Autodesk Inventor part; units mm, degrees
ref_plane "Arbeitsebene1" through (0, 0, 0) normal (0, 1, 0) x (-1, 0, 0)
ref_plane "YZ Plane" through (0, 0, 0) normal (1, 0, 0) x (0, 1, 0)
ref_plane "XY Plane" through (0, 0, 0) normal (0, 0, 1) x (1, 0, 0)
sketch "Skizze1" plane through (0, 0, 0) normal (0, 1, 0) x (-1, 0, 0)
  circle A0 centre (0, 0) radius 75
  dimension "d0" = 150
extrude "Extrusion1" add sketch "Skizze1" along normal mid plane 6
ref_plane "Arbeitsebene1" through (0, 0, 0) normal (0, 1, 0) x (-1, 0, 0)
sketch "Skizze4" plane through (0, 0, 0) normal (0, 1, 0) x (-1, 0, 0)
  circle A0 centre (0, 0) radius 6.5
  dimension "d17" = 13
extrude "Extrusion3" add sketch "Skizze4" along normal mid plane 18
sketch "Skizze5" plane through (0, 9, 0) normal (0, 1, 0) x (1, 0, 0)
  circle A0 centre (0, 0) radius 6.5
hole "Bohrung1" at (0, 9, 0) direction (0, -1, 0) diameter 6 end up to surface
sketch "Skizze2" plane through (0, 3, 0) normal (0, 1, 0) x (1, 0, 0)
  circle A0 centre (0, 0) radius 63 construction
  circle A1 centre (0, 0) radius 75
  line L0 (0, 0) -> (0, -75) construction
  line L1 (0, 0) -> (-75, 0) construction
  circle A2 centre (0, 0) radius 6.5
  line L2 (-8, 0) -> (-54.1014, -32.2806)
  line L3 (-8, 0) -> (-54.1014, 32.2806)
  arc A3 (-54.1014, 32.2806) -> (-54.1014, -32.2806) centre (0, 0) ccw
  dimension "d3" = 126
  dimension "d40" = 8
  dimension "d41" = 35
extrude "Extrusion2" cut sketch "Skizze2" against normal up to surface (6 mm away) contours L2 A3 L3
fillet "Rundung1" radius 3 3 edges at (-8, 0, 0) (-54.1014, 0, 32.2806) (-54.1014, 0, -32.2806)
pattern_circular "Runde Anordnung3" count 5 over 360 about axis through (0, 0, 0) along (0, 1, 0) of "Extrusion2"
fillet "Rundung3" radius 3 6 edges at (24.7949, 0, -57.9156) (62.743, 0, -5.6845) (62.743, 0, 5.6845) (24.7949, 0, 57.9156) (13.9824, 0, 61.4288) (-47.4189, 0, 41.4783)
properties part number "wheel" material "Aluminium 6061"
Build history of the part. All positions in model axes, mm. Round coordinates to 2 decimals unless told otherwise and drop trailing zeros. Write each loop counter-clockwise with the first axis right and the second up, starting at its lowest first coordinate (ties: lowest second). Pieces come first, ordered by that corner, then holes. Notation, with made-up numbers: (83, 7) -> (121, 7) arc R20 cw to (121, 36) -> close; hole circle Ø6 at (-13.5, 45). An arc over 180 degrees is marked (long way). Put each result on its own line as item: value.
Item 1: Slice it at B-B, the plane x = 0. Give the cut face in (y, z), plus the area to 3 significant figures.
Here are the results:
outline: (-9, -6.5) -> (-3, -6.5) -> (-3, -15.69) -> (3, -15.69) -> (3, -6.5) -> (9, -6.5) -> (9, -3) -> (-9, -3) -> close; (-9, 3) -> (9, 3) -> (9, 6.5) -> (3, 6.5) -> (3, 15.69) -> (-3, 15.69) -> (-3, 6.5) -> (-9, 6.5) -> close; (-3, -75) -> (3, -75) -> (3, -63) -> (-3, -63) -> close; (-3, 63) -> (3, 63) -> (3, 75) -> (-3, 75) -> close
area: 380 mm^2
Item 2: Two-plate mould, pull along X, no slides. Class faces 1 (the face through (5.158, -5.958, -3.955)), 2 (the face through (-19.874, 0.042, 59.783)), 3 (the face through (1, 3, -16)): pulls with the +X half, pulls with the -X half, needs draft (parallel to the pull), parting line crosses it, or undercut.
Here are the results:
face 1: parting line crosses it
face 2: undercut
face 3: needs draft
Item 3: Flat gauge pins, fed straight in: P1, Ø4, axis at x = -56, y = -3.5, coming from the -Z side; P2, Ø12, axis at x = -27, z = -53.5, coming from the +Y side. Where does each tip first touch, or does it go through?
Here are the results:
P1: stops at z = -51.98
P2: stops at y = 3
Item 4: Slice it at A-A, the plane z = 0. Give the cut face in (x, y).
Here are the results:
outline: (-75, -3) -> (-63, -3) -> (-63, 3) -> (-75, 3) -> close; (-10.23, -3) -> (-6.5, -3) -> (-6.5, -9) -> (-3, -9) -> (-3, 9) -> (-6.5, 9) -> (-6.5, 3) -> (-10.23, 3) -> close; (3, -9) -> (6.5, -9) -> (6.5, -3) -> (75, -3) -> (75, 3) -> (6.5, 3) -> (6.5, 9) -> (3, 9) -> close
Item 5: Slice it at C-C, the plane z = -49. Give the cut face in (x, y), plus the area to 3 significant figures.
Here are the results:
outline: (-56.78, -3) -> (-39.6, -3) -> (-39.6, 3) -> (-56.78, 3) -> close; (10.18, -3) -> (21.73, -3) -> (21.73, 3) -> (10.18, 3) -> close; (39.6, -3) -> (56.78, -3) -> (56.78, 3) -> (39.6, 3) -> close
area: 275 mm^2
Item 6: Wall check: probe 1 along Z at (x, y) = (0, -5); probe 2 along X at (y, z) = (-1.5, 2); probe 3 along Z at (x, y) = (-17, -0.25). Give the ranges that are in metal, low to high. Write a range as from..to.
Here are the results:
probe 1: z = -6.5..-3, 3..6.5
probe 2: x = -74.97..-62.97, -10.99..-2.24, 2.24..74.97
probe 3: z = -73.05..-60.66, -18.56..-6.3, 6.3..18.56, 60.66..73.05
Item 7: Slice it at D-D, the plane x = -41.5. Give the cut face in (y, z).
Here are the results:
outline: (-3, -62.47) -> (3, -62.47) -> (3, -47.4) -> (-3, -47.4) -> close; (-3, -37.02) -> (3, -37.02) -> (3, -23.46) -> (-3, -23.46) -> close; (-3, 23.46) -> (3, 23.46) -> (3, 37.02) -> (-3, 37.02) -> close; (-3, 47.4) -> (3, 47.4) -> (3, 62.47) -> (-3, 62.47) -> close
